Can you work these out from the model? Positions are in its coordinate system, mm. A direction names the side the tool comes from. Give positions to 0.01 mm unless a question says otherwise; leave off trailing zeros. Write each loop counter-clockwise with the first axis right and the second up, starting at its lowest first coordinate (ties: lowest second). Pieces come first, ordered by that corner, then holes.
```python
from build123d import *

# Parameters (mm, degrees)
F0_W           = 65
F0_H           = 36
F0_R           = 11.5
F1_DEPTH       = 6
F3_D           = 3.3
F3_CBORE_D     = 6.5
F3_CBORE_DEPTH = 3
F4_SIZE        = 0.5
F6_D           = 3.3
F6_CBORE_D     = 6.5
F6_CBORE_DEPTH = 3


with BuildPart() as f1:
    # F0 (on Front) → F1 (new body)
    with BuildSketch(Plane.XZ):
        Rectangle(F0_W, F0_H)
        Circle(F0_R, mode=Mode.SUBTRACT)
    extrude(amount=F1_DEPTH)

    # F3 (through all)
    with Locations(Plane.XZ.offset(6)):
        with Locations((13, 13), (13, -13), (-13, -13), (-13, 13)):
            CounterBoreHole(F3_D / 2, F3_CBORE_D / 2, F3_CBORE_DEPTH)

    # F4
    f4_edges = [f1.edges().sort_by_distance(p)[0] for p in [
        (-32.5, -3, 18),
        (32.5, -3, 18),
        (32.5, -3, -18),
        (-32.5, -3, -18),
    ]]
    chamfer(f4_edges, length=F4_SIZE)

    # F6 (through all)
    with Locations(Plane(origin=(0, 0, 0), x_dir=(-1, 0, 0), z_dir=(0, 1, 0))):
        with Locations((-27, -15), (27, -15)):
            CounterBoreHole(F6_D / 2, F6_CBORE_D / 2, F6_CBORE_DEPTH)


solid = f1.part
```
1) Suppose I cut it at C-C on y = -4.55. Write out the boundary of the cut face in (x, z).
Values follow:
outline: (-32.5, -17.5) - (-32, -18) - (32, -18) - (32.5, -17.5) - (32.5, 17.5) - (32, 18) - (-32, 18) - (-32.5, 17.5) - close; hole circle Ø3.3 at (-27, -15); hole circle Ø6.5 at (-13, -13); hole circle Ø6.5 at (-13, 13); hole circle Ø23 at (0, 0); hole circle Ø6.5 at (13, -13); hole circle Ø6.5 at (13, 13); hole circle Ø3.3 at (27, -15)
2) Suppose I cut it at B-B on z = 13. Write out the boundary of the cut face in (x, y).
Values follow:
outline: (-32.5, -6) - (-16.25, -6) - (-16.25, -3) - (-14.65, -3) - (-14.65, 0) - (-32.5, 0) - close; (-11.35, -3) - (-9.75, -3) - (-9.75, -6) - (9.75, -6) - (9.75, -3) - (11.35, -3) - (11.35, 0) - (-11.35, 0) - close; (14.65, -3) - (16.25, -3) - (16.25, -6) - (32.5, -6) - (32.5, 0) - (14.65, 0) - close
3) If we mould it in two halves opening along X, with no side actions, what happens to faces 4 (the face through (0, -3, 18)), 5 (the face through (10.605, -4.521, -10.803)), 6 (the face through (32.5, -3, 0))? For each: +X half, -X half, draft (parallel to the pull), parting line (faces both ways), or undercut.
Values follow:
face 4: draft
face 5: undercut
face 6: +X half
4) Suppose I cut it at A-A on x = 0. Write out the boundary of the cut face in (y, z), plus the area to 3 significant figures.
Values follow:
outline: (-6, -18) - (0, -18) - (0, -11.5) - (-6, -11.5) - close; (-6, 11.5) - (0, 11.5) - (0, 18) - (-6, 18) - close
area: 78.0 mm2
5) For pin 1 Ø2 at (x, z) = (13, -13) entering from -Y; pin 2 Ø2 at (x, z) = (-14.5, 12.5) entering from -Y; pin 3 Ø6 at (x, z) = (-27, -15) entering from +Y, each with a flat end and sliding along its axis, tell me the tip position at first contact or that it passes through.
Values follow:
pin 1: passes through
pin 2: stops at y = -3
pin 3: stops at y = -3
6) Suppose I cut it at D-D on y = -0.95. Write out the boundary of the cut face in (x, z).
Values follow:
outline: (-32.5, -17.5) - (-32, -18) - (-28.25, -18) arc R3.25 cw (long way) to (-25.75, -18) - (25.75, -18) arc R3.25 cw (long way) to (28.25, -18) - (32, -18) - (32.5, -17.5) - (32.5, 17.5) - (32, 18) - (-32, 18) - (-32.5, 17.5) - close; hole circle Ø3.3 at (-13, -13); hole circle Ø3.3 at (-13, 13); hole circle Ø23 at (0, 0); hole circle Ø3.3 at (13, -13); hole circle Ø3.3 at (13, 13)
7) For faces 1 (the face through (-11.6, -3, 11.6)), 2 (the face through (26.875, -1.479, -11.752)), 3 (the face through (-1.5, -3, 11.4)), which set-ups out of +Z, -Z, +X, -X, +Y, -Y let a thin tool reach every point of the face, with its end or its side?
Values follow:
face 1: -Y
face 2: +Y
face 3: +Y, -Y
8) Please list where these lines run through material, in increasing order: L1, parallel to X at y = -0.9, z = -15; L2, parallel to Z at x = -13, y = -5; L3, parallel to Z at x = 13, y = -1.2.
Values follow:
L1: x = -32.5 to -30.25, -23.75 to 23.75, 30.25 to 32.5
L2: z = -18 to -16.25, -9.75 to 9.75, 16.25 to 18
L3: z = -18 to -14.65, -11.35 to 11.35, 14.65 to 18
